```python
from build123d import *

# Parameters (mm, degrees)
F0_R      = 10.95
F0_R_2    = 0.069
F3_DEPTH  = 2
F1_R      = 5.5
F4_DEPTH  = 3
F2_R      = 4.025
F5_DEPTH  = 6
F6_R      = 0.5
F7_R      = 2.925
F8_DEPTH  = 4
F9_R      = 9.395345
F9_R_2    = 8.971159
F9_R_3    = 8.061351
F9_R_4    = 7.523244
F9_R_5    = 6.602201
F9_R_6    = 6.105505
F9_R_7    = 5.163827
F9_R_8    = 4.615079
F9_R_9    = 3.850939
F9_R_10   = 3.383897
F9_R_11   = 2.709612
F9_R_12   = 2.365196
F9_R_13   = 1.847375
F9_R_14   = 1.387714
F10_DEPTH = 1


with BuildPart() as f3:
    # F0 (on Top) → F3 (new body)
    with BuildSketch(Plane.XY):
        Circle(F0_R)
        Circle(F0_R_2, mode=Mode.SUBTRACT)
    extrude(amount=F3_DEPTH)

    # F1 (on Top) → F4 (join)
    with BuildSketch(Plane.XY):
        Circle(F1_R)
    extrude(amount=F4_DEPTH)

    # F2 (on Top) → F5 (join)
    with BuildSketch(Plane.XY):
        Circle(F2_R)
    extrude(amount=F5_DEPTH)

    # F6
    f6_edges = [f3.edges().sort_by_distance(p)[0] for p in [
        (10.95, 0, 1),
        (-10.95, 0, 0),
        (-10.95, 0, 2),
    ]]
    fillet(f6_edges, radius=F6_R)

    # F7 (on face) → F8 (cut)
    with BuildSketch(Plane.XY.offset(6)):
        Circle(F7_R)
    extrude(amount=-F8_DEPTH, mode=Mode.SUBTRACT)

    # F9 (on face) → F10 (cut)
    with BuildSketch(Plane(origin=(0, 0, 0), x_dir=(1, 0, 0), z_dir=(0, 0, -1))):
        Circle(F9_R)
        Circle(F9_R_2, mode=Mode.SUBTRACT)
        Circle(F9_R_3)
        Circle(F9_R_4, mode=Mode.SUBTRACT)
        Circle(F9_R_5)
        Circle(F9_R_6, mode=Mode.SUBTRACT)
        Circle(F9_R_7)
        Circle(F9_R_8, mode=Mode.SUBTRACT)
        Circle(F9_R_9)
        Circle(F9_R_10, mode=Mode.SUBTRACT)
        Circle(F9_R_11)
        Circle(F9_R_12, mode=Mode.SUBTRACT)
        Circle(F9_R_13)
        Circle(F9_R_14, mode=Mode.SUBTRACT)
    extrude(amount=-F10_DEPTH, mode=Mode.SUBTRACT)


solid = f3.part
```
Geometry: final body of the model. Coordinates: model frame, mm. A direction names the side the tool comes from. Give positions to 0.01 mm unless a question says otherwise; leave off trailing zeros. Write each loop counter-clockwise with the first axis right and the second up, starting at its lowest first coordinate (ties: lowest second). Pieces come first, ordered by that corner, then holes.
1. Pin query (flat end, axial travel): P1, Ø4.5, axis at x = 0, y = 0, coming from the +Z side; P2, Ø10, axis at x = -6.5, y = -7, coming from the +Z side; P3, Ø1.5, axis at x = -0.5, z = 4, coming from the +Y side (3 decimals); P4, Ø1.5, axis at x = -7, z = 3, coming from the +Y side. Return the tip coordinate at first contact, or that it passes through.
2. Section query A-A, the plane z = 3.3. Return loops of the section in (x, y) (3 decimals).
3. Line query: probe 1 along Z at (x, y) = (5.5, 1.5); probe 2 along X at (y, z) = (-2, 5.7); probe 3 along Z at (x, y) = (-3, -2.75). Output: solid intervals per line, ascending.
4. Reachability of faces 4 (the cylindrical face through (-0.4, 1.803, 0.493)), 5 (the flat face through (4, -4, 2)), 6 (the flat face through (-9, 4, 0)) from +Z, -Z, +X, -X, +Y, -Y: full face, straight path, thin tool, end or side. Return the list, or none.
5. Draft query along X for faces 1 (the flat face through (-5, 3, 0)), 2 (the cylindrical face through (-1.19, -5.37, 2.49)), 3 (the cylindrical face through (-1, 4.505, 0.493)). Return one class per face: released by +X, released by -X, zero draft, split by the parting line, or undercut.
Computed:
1. P1: stops at z = 2
1. P2: stops at z = 3
1. P3: stops at y = 4.025
1. P4: passes through
2. outline: circle Ø8.05 at (0, 0); hole circle Ø5.85 at (0, 0)
3. probe 1: z = 0 to 2
3. probe 2: x = -3.49 to -2.13, 2.13 to 3.49
3. probe 3: z = 0 to 3
4. face 4: -Z
4. face 5: +Z
4. face 6: -Z, +X, -X, +Y, -Y
5. face 1: zero draft
5. face 2: split by the parting line
5. face 3: undercut
